Can you work these out from the drawing? Everything is in mm from the part's minimum corner. A direction names the side the tool comes from. Round coordinates to 2 decimals unless told otherwise and drop trailing zeros. Order: outer loops, then holes, each group sorted by start corner. A loop starts at its lowest first (then second) coordinate and runs counter-clockwise, first axis right, second up. Notation, with made-up numbers: (78, -39.75) - (85, -39.75) arc R17 cw to (85, -15.75) - close; hole circle Ø5 at (25.5, 3). An arc over 180 degrees is marked (long way). Answer as a JSON object with one key per item and string values.
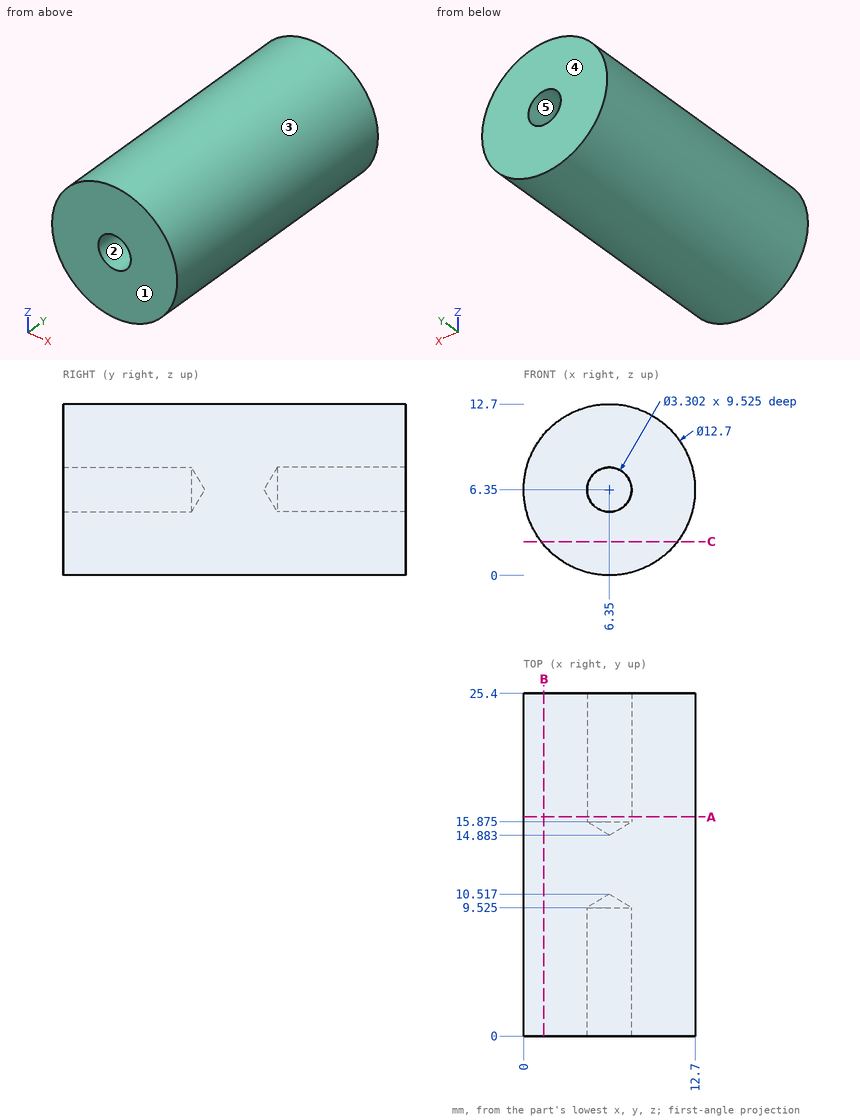
1. Imagine slicing it at B-B (x = 1.5). List the corners of the cut face in (y, z) for me.
Responses:
{"outline": "(0, 2.25) - (25.4, 2.25) - (25.4, 10.45) - (0, 10.45) - close"}
2. If I drill on L1, parallel to Z at x = 6.35, y = 7; L2, parallel to X at y = 8.5, z = 6.5; L3, parallel to X at y = 9.5, z = 2.25, over which ranges is the centre line in solid material (lowest first)? Write a range as [from, to].
Responses:
{"L1": "[0, 4.7], [8, 12.7]", "L2": "[0, 4.71], [7.99, 12.7]", "L3": "[1.5, 11.2]"}
3. Thinking about a two-plate mould opening in X: for the marked faces 1, 2 and 3, which applies, pulls with the +X half, pulls with the -X half, needs draft (parallel to the pull), parting line crosses it, or undercut?
Responses:
{"face 1": "needs draft", "face 2": "undercut", "face 3": "parting line crosses it"}
4. Imagine slicing it at C-C (z = 2.5). List the corners of the cut face in (x, y) for me, plus the area to 3 significant figures.
Responses:
{"outline": "(1.3, 0) - (11.4, 0) - (11.4, 25.4) - (1.3, 25.4) - close", "area": "257 mm2"}
5. Imagine slicing it at A-A (y = 16.25). List the corners of the cut face in (x, z) for me, plus the area to 3 significant figures.
Responses:
{"outline": "circle Ø12.7 at (6.35, 6.35); hole circle Ø3.3 at (6.35, 6.35)", "area": "118 mm2"}
6. For P1, Ø1, axis at x = 5.5, y = 16, coming from the +Z side; P2, Ø2, axis at x = 6.35, z = 6.35, coming from the +Y side; P3, Ø3, axis at x = 4, y = 11.5, coming from the +Z side, each with a flat end and sliding along its axis, tell me the tip position at first contact or that it passes through.
Responses:
{"P1": "z = 12.69", "P2": "y = 15.48", "P3": "z = 12.64"}
7. For the marked faces 4 and 5, which set-ups out of +Z, -Z, +X, -X, +Y, -Y let a thin tool reach every point of the face, with its end or its side?
Responses:
{"face 4": "+Z, -Z, +X, -X, +Y", "face 5": "+Y"}
